from build123d import *

# Parameters (mm, degrees)
F0_R     = 12.25
F0_R_2   = 1.8
F0_R_3   = 4.65
F1_DEPTH = 10
F2_SIZE  = 1.5
F3_SIZE  = 0.49999


# Not quite as in the source:
# - a fillet or chamfer is up to 0.001 mm smaller than in the source, because OpenCascade refuses the exact size


with BuildPart() as f1:
    # F0 (on Top) → F1 (new body)
    with BuildSketch(Plane.XY):
        Circle(F0_R)
        with Locations((0, -8.45)):
            Circle(F0_R_2, mode=Mode.SUBTRACT)
        with Locations((-8.45, 0)):
            Circle(F0_R_2, mode=Mode.SUBTRACT)
        Circle(F0_R_3, mode=Mode.SUBTRACT)
        with Locations((8.45, 0)):
            Circle(F0_R_2, mode=Mode.SUBTRACT)
        with Locations((0, 8.45)):
            Circle(F0_R_2, mode=Mode.SUBTRACT)
    extrude(amount=F1_DEPTH)

    # F2
    f2_edges = [f1.edges().sort_by_distance(p)[0] for p in [
        (-10.25, 0, 10),
        (-1.8, 8.45, 10),
        (6.65, 0, 10),
        (-1.8, -8.45, 10),
    ]]
    chamfer(f2_edges, length=F2_SIZE)

    # F3 (size 0.5 in the source; OpenCascade refuses exactly that, so slightly less here)
    f3_edges = [f1.edges().sort_by_distance(p)[0] for p in [
        (-4.65, 0, 10),
    ]]
    chamfer(f3_edges, length=F3_SIZE)


solid = f1.part
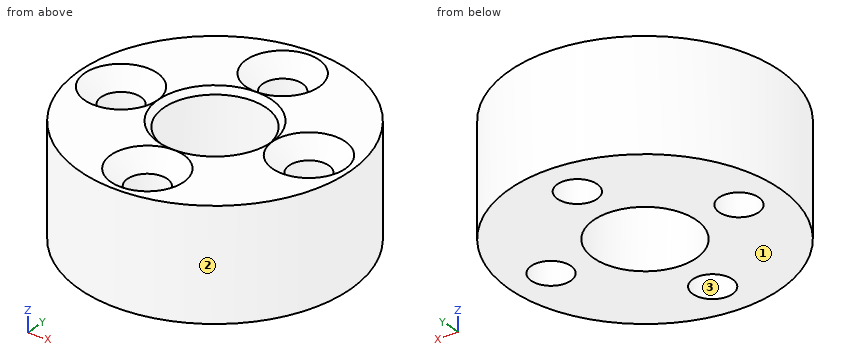
Can you work these out from the model? Positions are in its coordinate system, mm. Face numbers are marked on the shaded views. Coordinates: 2 decimals unless noted, no trailing zeros. Loops run counter-clockwise (first coordinate to the right, second up) from the corner with the lowest first, then second, coordinate; pieces in that order, holes last. Notation, with made-up numbers: (10.5, 52.5) - (33.5, 52.5) arc R36 cw to (33.5, 91.5) - close; hole circle Ø7 at (-13, 39). An arc over 180 degrees is marked (long way). Answer as a JSON object with one key per item and string values. Group by question number.
Item 1: If we section it at C-C (z = 1.5): List the corners of the cut face in (x, y) for me, plus the area to 3 significant figures.
Item 2: For pin 1 (2 mm diameter, centred on y = 7.5, z = 5, fed in from -X); pin 2 (4 mm diameter, centred on x = 0, y = 8.45, fed in from +Z); pin 3 (1 mm diameter, centred on y = -7, z = 6.5, fed in from +X), each with a flat end and sliding along its axis, tell me the tip position at first contact or that it passes through.
Item 3: If we section it at A-A (y = 0): State how many separate pieces and enclosed holes the cut face has, plus the area to 4 significant figures.
Item 4: If we mould it in two halves opening along X, with no side actions, what happens to the marked faces 1, 2 and 3? For each: released by +X, released by -X, zero draft, split by the parting line, or undercut.
Item 5: If I drill on L1, parallel to Y at x = 0, z = 7; L2, parallel to X at y = 7, z = 6.5; L3, parallel to X at y = 1, z = 9, over which ranges is the centre line in solid material (lowest first)? Write a range as from..to.
Item 6: If we section it at B-B (x = -8.45): List the corners of the cut face in (y, z) for me, plus the area to 3 significant figures.
Returned:
{
 "1": {"outline": "circle Ø24.5 at (0, 0); hole circle Ø3.6 at (-8.45, 0); hole circle Ø9.3 at (0, 0); hole circle Ø3.6 at (0, -8.45); hole circle Ø3.6 at (0, 8.45); hole circle Ø3.6 at (8.45, 0)", "area": "363 mm²"},
 "2": {"pin 1": "stops at x = -10.38", "pin 2": "stops at z = 8.7", "pin 3": "stops at x = 10.38"},
 "3": {"separate pieces": "4", "enclosed holes": "0", "area": "75.25 mm²"},
 "4": {"face 1": "zero draft", "face 2": "split by the parting line", "face 3": "undercut"},
 "5": {"L1": "y = -12.25..-10.25, -6.65..-4.65, 4.65..6.65, 10.25..12.25", "L2": "x = -10.05..-1.07, 1.07..10.05", "L3": "x = -12.21..-10.52, -6.38..-4.54, 4.54..6.38, 10.52..12.21"},
 "6": {"outline": "(-8.87, 0) - (-1.8, 0) - (-1.8, 8.5) - (-3.3, 10) - (-8.87, 10) - close; (1.8, 0) - (8.87, 0) - (8.87, 10) - (3.3, 10) - (1.8, 8.5) - close", "area": "139 mm²"}
}
